The listing builds one solid part. Answer for the finished solid, in the listing's coordinates (mm). Face numbers are marked on the shaded views. A direction names the side the tool comes from. Coordinates: 2 decimals unless noted, no trailing zeros. Order: outer loops, then holes, each group sorted by start corner. A loop starts at its lowest first (then second) coordinate and runs counter-clockwise, first axis right, second up. Notation, with made-up numbers: (71, 25) -> (77, 25) arc R11 ccw to (77, 40) -> close; hole circle Ø10 at (-32.5, 56.25). An arc over 180 degrees is marked (long way). Write each question's results on one line, items separated by ' | '. Start each with the question number.
(1) Determine the mould class of the marked faces 1, 2 and 3 for opening direction X: +X half, -X half, draft (parallel to the pull), parting line (faces both ways), or undercut.
(2) Straight lines are drawn through the part: L1, parallel to Z at x = -42, y = 40; L2, parallel to Y at x = -35, z = 12.5; L3, parallel to Y at x = 18, z = -13.5. For each, find the intervals that lie inside material, in ascending order.
(3) The part is cut by section D-D, the plane x = -32. Give the vertices of the cut face in (y, z), then the cut area to 3 significant figures.
(4) Given pin 1 (12 mm diameter, centred on y = 11.5, z = -12, fed in from +X); pin 2 (8 mm diameter, centred on x = 24, y = 13, fed in from +Z); pin 3 (2.5 mm diameter, centred on y = 20, z = -15, fed in from +X); pin 4 (6.5 mm diameter, centred on y = 12, z = 15.5, fed in from +X), each flat-ended and moving along its own axis, determine where each tip first touches the part or whether it passes through.
(5) The part is cut by section B-B, the plane z = 14. Give the vertices of the cut face in (x, y) (3 decimals), then the cut area to 3 significant figures.
(6) A tool of negligible diameter and unlimited length cuts with its end or side. For the marked faces 4 and 5, from which of +Z, -Z, +X, -X, +Y, -Y can it reach the whole face along a straight path? Write none if from no direction.
(7) The part is cut by section A-A, the plane y = 8. Give the vertices of the cut face in (x, z).
(8) The part is cut by section C-C, the plane y = 21.5. Give the vertices of the cut face in (x, z), then the cut area to 3 significant figures.
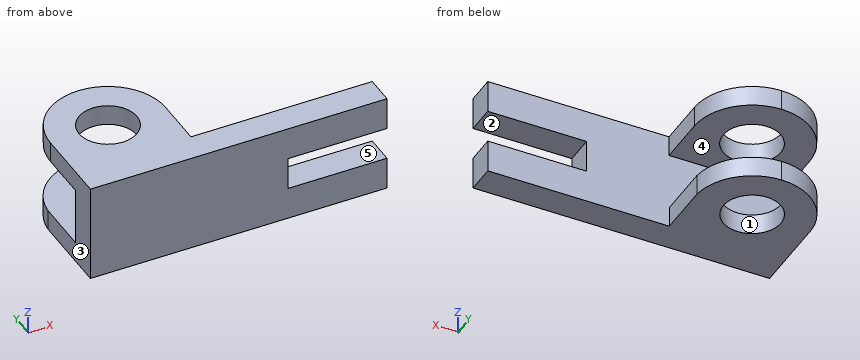
```python
from build123d import *

# Parameters (mm, degrees)
SKETCH1_W           = 114.3
SKETCH1_H           = 11.1125
BOSS_EXTRUDE1_DEPTH = 19.05
SKETCH3_W           = 12.7
SKETCH3_H           = 11.1125
CUT_EXTRUDE1_DEPTH  = 38.1
SKETCH4_R           = 11.115
BOSS_EXTRUDE2_DEPTH = 7.9375
SKETCH5_R           = 11.1125
BOSS_EXTRUDE3_DEPTH = 7.9375


with BuildPart() as part:
    # Sketch1 → Boss-Extrude1 (new, symmetric)
    with BuildSketch(Plane.XY):
        Rectangle(SKETCH1_W, SKETCH1_H)
    extrude(amount=BOSS_EXTRUDE1_DEPTH, both=True)

    # Sketch3 → Cut-Extrude1 (cut)
    with BuildSketch(Plane(origin=(57.15, 0, 0), x_dir=(0, 0, -1), z_dir=(1, 0, 0))):
        Rectangle(SKETCH3_W, SKETCH3_H)
    extrude(amount=-CUT_EXTRUDE1_DEPTH, mode=Mode.SUBTRACT)

    # Sketch4 → Boss-Extrude2 (add)
    with BuildSketch(Plane.XY.offset(19.05)):
        with BuildLine():
            Line((-57.15, 24.60625), (-57.15, 5.55625))
            Line((-57.15, 5.55625), (-12.7, 5.55625))
            Line((-12.7, 5.55625), (-12.7, 24.60625))
            ThreePointArc((-12.7, 24.60625), (-19.209551788, 40.321698212), (-34.925, 46.83125))
            ThreePointArc((-34.925, 46.83125), (-50.640448212, 40.321698212), (-57.15, 24.60625))
        make_face()
        with Locations((-34.925, 24.60625)):
            Circle(SKETCH4_R, mode=Mode.SUBTRACT)
    extrude(amount=-BOSS_EXTRUDE2_DEPTH)

    # Sketch5 → Boss-Extrude3 (add)
    with BuildSketch(Plane(origin=(0, 0, -19.05), x_dir=(-1, 0, 0), z_dir=(0, 0, -1))):
        with BuildLine():
            Line((12.804049861, 5.55625), (57.15, 5.55625))
            Line((57.15, 5.55625), (57.15, 26.195))
            ThreePointArc((57.15, 26.195), (50.122971728, 40.875602864), (34.977024762, 46.83375))
            ThreePointArc((34.977024762, 46.83375), (19.83107801, 40.875602749), (12.804049861, 26.195))
            Line((12.804049861, 26.195), (12.804049861, 5.55625))
        make_face()
        with Locations((34.97702493, 24.60375)):
            Circle(SKETCH5_R, mode=Mode.SUBTRACT)
    extrude(amount=-BOSS_EXTRUDE3_DEPTH)


solid = part.part
```
Established:
1) face 1: undercut | face 2: draft | face 3: -X half
2) L1: z = -19.05 to -11.11, 11.11 to 19.05 | L2: y = -5.56 to 13.49, 35.72 to 46.83 | L3: y = -5.56 to 5.56
3) outline: (-5.56, -19.05) -> (13.9, -19.05) -> (13.9, -11.11) -> (5.56, -11.11) -> (5.56, 11.11) -> (13.88, 11.11) -> (13.88, 19.05) -> (-5.56, 19.05) -> close; (35.31, -19.05) -> (46.63, -19.05) -> (46.63, -11.11) -> (35.31, -11.11) -> close; (35.33, 11.11) -> (46.64, 11.11) -> (46.64, 19.05) -> (35.33, 19.05) -> close | area: 735 mm^2
4) pin 1: stops at x = 57.15 | pin 2: passes through | pin 3: stops at x = -12.8 | pin 4: stops at x = -12.7
5) outline: (-57.15, -5.556) -> (57.15, -5.556) -> (57.15, 5.556) -> (-12.7, 5.556) -> (-12.7, 24.606) arc R22.225 ccw to (-57.15, 24.606) -> close; hole circle Ø22.23 at (-34.925, 24.606) | area: 2,500 mm^2
6) face 4: +X, -X, +Y | face 5: +X, +Y, -Y
7) outline: (-57.15, -19.05) -> (-12.8, -19.05) -> (-12.8, -11.11) -> (-57.15, -11.11) -> close; (-57.15, 11.11) -> (-12.7, 11.11) -> (-12.7, 19.05) -> (-57.15, 19.05) -> close
8) outline: (-57.15, -19.05) -> (-45.65, -19.05) -> (-45.65, -11.11) -> (-57.15, -11.11) -> close; (-57.15, 11.11) -> (-45.6, 11.11) -> (-45.6, 19.05) -> (-57.15, 19.05) -> close; (-24.31, -19.05) -> (-12.8, -19.05) -> (-12.8, -11.11) -> (-24.31, -11.11) -> close; (-24.25, 11.11) -> (-12.7, 11.11) -> (-12.7, 19.05) -> (-24.25, 19.05) -> close | area: 366 mm^2
